Design review of the part built by this model. Coordinates are the model's own, in mm. A direction names the side the tool comes from. Coordinates: 2 decimals unless noted, no trailing zeros. Loops run counter-clockwise (first coordinate to the right, second up) from the corner with the lowest first, then second, coordinate; pieces in that order, holes last. Notation, with made-up numbers: M 64.25,43 L 79.25,43 A20 ccw 79.25,68 Z; hole C 2,81.5 d2. An arc over 180 degrees is marked long. Put each result on its own line as item: value. Start each with the question number.
(1) Clearance check with flat-ended pins moving along their axes: pin 1 (2 mm diameter, centred on x = 3.5, z = 13, fed in from +Y); pin 2 (3 mm diameter, centred on x = -0.5, y = -1.5, fed in from +Z); pin 3 (5 mm diameter, centred on y = -14.5, z = 14, fed in from -X). State where each tip first meets the part, or that it passes through.
(2) For probe 1 along Y at (x, z) = (0, 7); probe 2 along Y at (x, z) = (-0.5, 16.25); probe 3 along X at (y, z) = (0.5, 4), list the stretches that pass through material, from the lowest coordinate up. Write a range as [from, to].
(3) Take a section at C-C, the plane y = 0. Give the boundary of the cut face in (x, z), then the cut area to 3 significant figures.
(4) Take a section at B-B, the plane z = 15. Give the boundary of the cut face in (x, y), then the cut area to 3 significant figures.
(5) Take a section at D-D, the plane x = 0. Give the boundary of the cut face in (y, z).
(6) Take a section at A-A, the plane z = 10.25. Give the boundary of the cut face in (x, y).
(7) The part is to be moulded in two halves that separate along X. For faces 3 (the flat face through (0, 0, 0)), 4 (the cylindrical face through (-4.336, -19.524, 9.134)), 5 (the cylindrical face through (-13.887, -10.648, 10.148)), say which applies: +X half, -X half, draft (parallel to the pull), parting line (faces both ways), or undercut.
(8) For faces 1 (the flat face through (-1, -1, 4.5)), 2 (the flat face through (0, -18, 17.5)), list the 3-axis set-ups (+Z, -Z, +X, -X, +Y, -Y) from which the entire face can be reached by the end or side of a thin tool; tool diameter is ignored.
```python
from build123d import *

# Parameters (mm, degrees)
SKETCH1_R           = 20
BOSS_EXTRUDE1_DEPTH = 15
SKETCH2_R           = 17.5
SKETCH2_R_2         = 5
CUT_EXTRUDE1_DEPTH  = 12
CUT_EXTRUDE2_DEPTH  = 10.5
SKETCH4_R           = 5
CUT_EXTRUDE3_DEPTH  = 1.5
CHAMFER1_SIZE       = 1
SKETCH7_R           = 20
SKETCH7_R_2         = 17.5
BOSS_EXTRUDE2_DEPTH = 2.5


with BuildPart() as part:
    # Sketch1 → Boss-Extrude1 (new body)
    with BuildSketch(Plane.XY):
        Circle(SKETCH1_R)
    extrude(amount=BOSS_EXTRUDE1_DEPTH)

    # Sketch2 → Cut-Extrude1 (cut)
    with BuildSketch(Plane.XY.offset(15)):
        Circle(SKETCH2_R)
        Circle(SKETCH2_R_2, mode=Mode.SUBTRACT)
    extrude(amount=-CUT_EXTRUDE1_DEPTH, mode=Mode.SUBTRACT)

    # Sketch3 → Cut-Extrude2 (cut)
    with BuildSketch(Plane.XY.offset(15)):
        with BuildLine():
            Line((-0.682606966, 3.228629389), (3.014916342, -1.341744927))
            ThreePointArc((3.014916342, -1.341744927), (-2.565540314, -2.075572908), (-0.682606966, 3.228629389))
        make_face()
    extrude(amount=-CUT_EXTRUDE2_DEPTH, mode=Mode.SUBTRACT)

    # Sketch4 → Cut-Extrude3 (cut)
    with BuildSketch(Plane.XY.offset(15)):
        Circle(SKETCH4_R)
    extrude(amount=-CUT_EXTRUDE3_DEPTH, mode=Mode.SUBTRACT)

    # Chamfer1
    chamfer1_edges = [part.edges().sort_by_distance(p)[0] for p in [
        (-20, 0, 0),
    ]]
    chamfer(chamfer1_edges, length=CHAMFER1_SIZE)

    # Sketch7 → Boss-Extrude2 (add)
    with BuildSketch(Plane.XY.offset(15)):
        Circle(SKETCH7_R)
        Circle(SKETCH7_R_2, mode=Mode.SUBTRACT)
    extrude(amount=BOSS_EXTRUDE2_DEPTH)


solid = part.part
```
Computed values:
1. pin 1: stops at y = 19.84
1. pin 2: stops at z = 4.5
1. pin 3: stops at x = -16
2. probe 1: y = [-20, -17.5], [-5, -3.3], [2.38, 5], [17.5, 20]
2. probe 2: y = [-19.99, -17.49], [17.49, 19.99]
2. probe 3: x = [-19.99, -17.49], [-4.97, 4.97], [17.49, 19.99]
3. outline: M -20,1 L -19,0 L 19,0 L 20,1 L 20,17.5 L 17.5,17.5 L 17.5,3 L 5,3 L 5,13.5 L 1.93,13.5 L 1.93,4.5 L -3.3,4.5 L -3.3,13.5 L -5,13.5 L -5,3 L -17.5,3 L -17.5,17.5 L -20,17.5 Z
3. area: 249 mm^2
4. outline: C 0,0 d40; hole C 0,0 d35
4. area: 295 mm^2
5. outline: M -20,1 L -19,0 L 19,0 L 20,1 L 20,17.5 L 17.5,17.5 L 17.5,3 L 5,3 L 5,13.5 L 2.38,13.5 L 2.38,4.5 L -3.3,4.5 L -3.3,13.5 L -5,13.5 L -5,3 L -17.5,3 L -17.5,17.5 L -20,17.5 Z
6. outline: C 0,0 d40; C 0,0 d10; hole C 0,0 d35; hole M -0.68,3.23 A3.3 ccw long 3.01,-1.34 Z
7. face 3: draft
7. face 4: parting line
7. face 5: undercut
8. face 1: +Z
8. face 2: +Z, +X, -X, +Y, -Y
